from build123d import *

# Parameters (mm, degrees)
SKETCH1_W           = 310
SKETCH1_H           = 280
SKETCH1_W_2         = 285
SKETCH1_H_2         = 255
BOSS_EXTRUDE1_DEPTH = 43
SKETCH2_W           = 20
SKETCH2_H           = 10
BOSS_EXTRUDE2_DEPTH = 25


with BuildPart() as part:
    # Sketch1 → Boss-Extrude1 (new body)
    with BuildSketch(Plane(origin=(0, 0, 0), x_dir=(1, 0, 0), z_dir=(0, 1, 0))):
        with Locations((155, 140)):
            Rectangle(SKETCH1_W, SKETCH1_H)
        with Locations((155, 140)):
            Rectangle(SKETCH1_W_2, SKETCH1_H_2, mode=Mode.SUBTRACT)
    extrude(amount=BOSS_EXTRUDE1_DEPTH)

    # Sketch2 → Boss-Extrude2 (add)
    with BuildSketch(Plane.ZY):
        with Locations((-218.75, 38)):
            Rectangle(SKETCH2_W, SKETCH2_H)
        with Locations((-31.25, 38)):
            Rectangle(SKETCH2_W, SKETCH2_H)
    extrude(amount=BOSS_EXTRUDE2_DEPTH)


solid = part.part
Verification items for the finished model (mm, model axes). A direction names the side the tool comes from. Round coordinates to 2 decimals unless told otherwise and drop trailing zeros. Loops run counter-clockwise (first coordinate to the right, second up) from the corner with the lowest first, then second, coordinate; pieces in that order, holes last. Notation, with made-up numbers: (89, -7.5) - (147, -7.5) arc R27 cw to (147, 17.5) - close; hole circle Ø5 at (-30, 60.25). An arc over 180 degrees is marked (long way). Use a Markdown table: item, result. Add a question column.
1. Thickness scan on probe 1 along X at (y, z) = (14, -107); probe 2 along Z at (x, y) = (138, 28); probe 3 along X at (y, z) = (31.5, -11). Record the ranges inside material, lowest first. Write a range as [from, to].
2. Section check A-A, the plane x = 109.5. Record the boundary of the cut face in (y, z).
3. Access from +Z, -Z, +X, -X, +Y, -Y to the whole of each face (thin tool, end or side, straight path). Record for faces 4 (the face through (-12, 38, -21.25)), 5 (the face through (-12, 38, -228.75)), 6 (the face through (-12, 38, -41.25)), 7 (the face through (297.5, 21, -138)).
4. Gauge pin test, flat ends, axial feed: pin 1 (3 mm diameter, centred on y = 13.5, z = -184.5, fed in from -X); pin 2 (3 mm diameter, centred on x = -12, y = 36.5, fed in from +Z); pin 3 (11 mm diameter, centred on x = -15, y = 40, fed in from -Z). Record the tip position at first contact, or that the pin passes through.
5. Section check B-B, the plane y = 21.5. Record the boundary of the cut face in (x, z).
6. Section check C-C, the plane z = -194. Record the boundary of the cut face in (x, y).
7. Release check for a two-part mould opening along X. For faces 1 (the face through (-25, 38, -219)), 2 (the face through (153, 21, -267.5)), 3 (the face through (-12, 33, -219)) record: released by +X, released by -X, zero draft, split by the parting line, or undercut.
Checks:
| question | item | result |
|---|---|---|
| 1 | probe 1 | x = [0, 12.5], [297.5, 310] |
| 1 | probe 2 | z = [-280, -267.5], [-12.5, 0] |
| 1 | probe 3 | x = [0, 310] |
| 2 | outline | (0, -280) - (43, -280) - (43, -267.5) - (0, -267.5) - close; (0, -12.5) - (43, -12.5) - (43, 0) - (0, 0) - close |
| 3 | face 4 | +Z, -X, +Y, -Y |
| 3 | face 5 | -Z, -X, +Y, -Y |
| 3 | face 6 | -X, +Y, -Y |
| 3 | face 7 | +Y, -Y |
| 4 | pin 1 | stops at x = 0 |
| 4 | pin 2 | stops at z = -21.25 |
| 4 | pin 3 | stops at z = -228.75 |
| 5 | outline | (0, -280) - (310, -280) - (310, 0) - (0, 0) - close; hole (12.5, -267.5) - (297.5, -267.5) - (297.5, -12.5) - (12.5, -12.5) - close |
| 6 | outline | (0, 0) - (12.5, 0) - (12.5, 43) - (0, 43) - close; (297.5, 0) - (310, 0) - (310, 43) - (297.5, 43) - close |
| 7 | face 1 | released by -X |
| 7 | face 2 | undercut |
| 7 | face 3 | zero draft |
